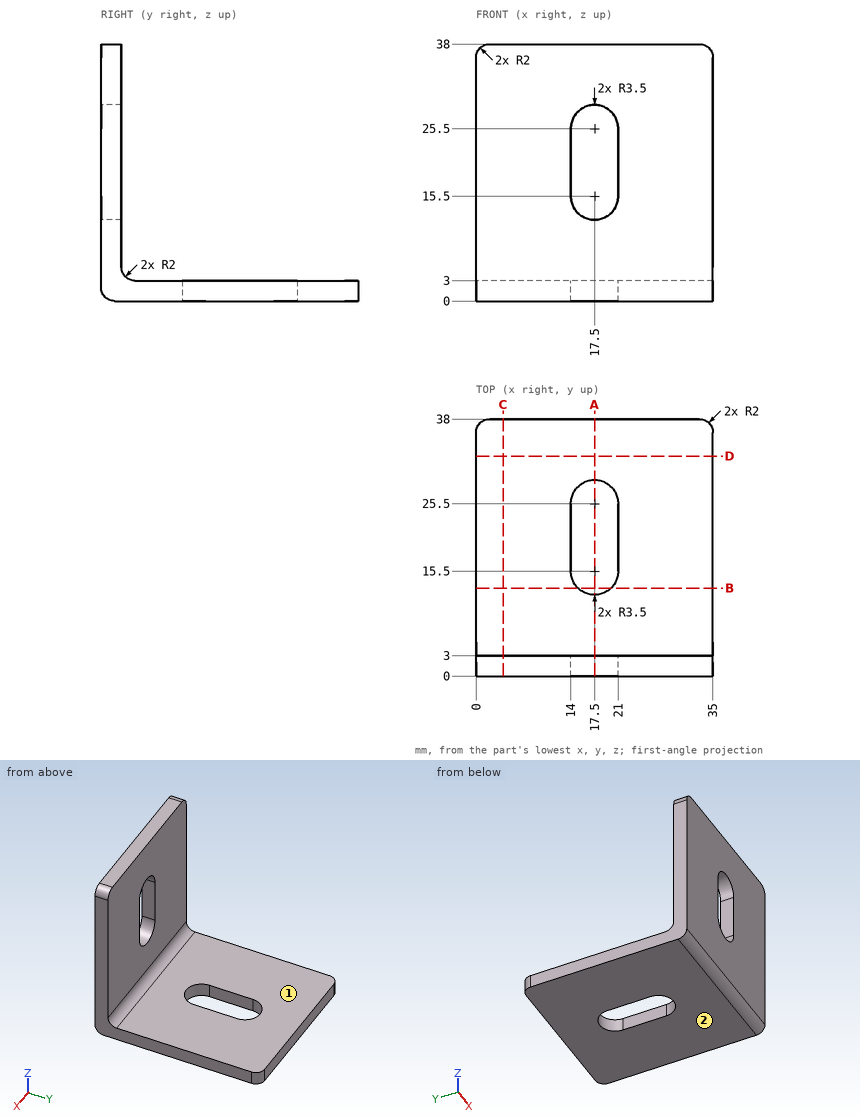
Print and shaded views of the part. All mm, measured from the part's lowest x, y and z. A direction names the side the tool comes from. Give positions to 0.01 mm unless a question says otherwise; leave off trailing zeros. Loops run counter-clockwise (first coordinate to the right, second up) from the corner with the lowest first, then second, coordinate; pieces in that order, holes last. Notation, with made-up numbers: (69, 81) - (85, 81) arc R13 ccw to (85, 91) - close; hole circle Ø3 at (-17.75, 52.25). An arc over 180 degrees is marked (long way). Use a Markdown table: item, result.
(1) Band-saw the part on A-A (x = 17.5). Give the cut face in (y, z), and give its area (3 significant figures).
Taken from the geometry:
| item | result |
|---|---|
| outline | (0, 2) arc R2 ccw to (2, 0) - (12, 0) - (12, 3) - (5, 3) arc R2 cw to (3, 5) - (3, 12) - (0, 12) - close; (0, 29) - (3, 29) - (3, 38) - (0, 38) - close; (29, 0) - (38, 0) - (38, 3) - (29, 3) - close |
| area | 117 mm2 |
(2) Wall check: line 1 along Y through (x, z) = (12.5, 12); line 2 along Y through (x, z) = (6.5, 4). Give the ranges that are in metal, low to high.
Taken from the geometry:
| item | result |
|---|---|
| line 1 | 0 to 3 |
| line 2 | 0 to 3.27 |
(3) Drop flat-ended pins along their axis: pin 1 Ø3 at (x, y) = (29, 9.5) entering from +Z; pin 2 Ø10 at (x, z) = (20.5, 24.5) entering from +Y. Give the stop position or say it passes through.
Taken from the geometry:
| item | result |
|---|---|
| pin 1 | z = 3 |
| pin 2 | y = 3 |
(4) Band-saw the part on B-B (y = 13). Give the cut face in (x, z), and give its area (3 significant figures).
Taken from the geometry:
| item | result |
|---|---|
| outline | (0, 0) - (15.05, 0) - (15.05, 3) - (0, 3) - close; (19.95, 0) - (35, 0) - (35, 3) - (19.95, 3) - close |
| area | 90.3 mm2 |
(5) Band-saw the part on C-C (x = 4). Give the cut face in (y, z), and give its area (3 significant figures).
Taken from the geometry:
| item | result |
|---|---|
| outline | (0, 2) arc R2 ccw to (2, 0) - (38, 0) - (38, 3) - (5, 3) arc R2 cw to (3, 5) - (3, 38) - (0, 38) - close |
| area | 219 mm2 |
(6) Which spindle directions (+Z, -Z, +X, -X, +Y, -Y) get a long thin tool onto all of the face, cutting with end or side? Do the marked faces 1 and 2. Say none if no direction does.
Taken from the geometry:
| item | result |
|---|---|
| face 1 | +Z, +X, -X, +Y |
| face 2 | -Z, +X, -X, +Y, -Y |
(7) Band-saw the part on D-D (y = 32.5). Give the cut face in (x, z), and give its area (3 significant figures).
Taken from the geometry:
| item | result |
|---|---|
| outline | (0, 0) - (35, 0) - (35, 3) - (0, 3) - close |
| area | 105 mm2 |
